```python
from build123d import *

# Parameters (mm, degrees)
F0_W     = 63.5
F0_H     = 63.5
F0_R     = 15.9639
F1_DEPTH = 19.05
F2_R     = 3.175
F3_DEPTH = 34.925


with BuildPart() as f1:
    # F0 (on Front) → F1 (new body, symmetric)
    with BuildSketch(Plane.XZ):
        Rectangle(F0_W, F0_H)
        Circle(F0_R, mode=Mode.SUBTRACT)
    extrude(amount=F1_DEPTH, both=True)

    # F2 (on Right) → F3 (cut, symmetric)
    with BuildSketch(Plane.YZ):
        with Locations((0, 22.225)):
            Circle(F2_R)
        with Locations((0, -22.225)):
            Circle(F2_R)
    extrude(amount=F3_DEPTH, both=True, mode=Mode.SUBTRACT)


solid = f1.part
```
Model file for the job. Use its own axes, mm. Coordinates: 2 decimals unless noted, no trailing zeros. Order: outer loops, then holes, each group sorted by start corner. A loop starts at its lowest first (then second) coordinate and runs counter-clockwise, first axis right, second up. Notation, with made-up numbers: (88, 17) -> (114, 17) arc R33 ccw to (114, 48) -> close; hole circle Ø5 at (51.5, -29.75). An arc over 180 degrees is marked (long way). Answer as a JSON object with one key per item and string values. Group by question number.
1) Pull direction Y, two halves, no side cores. Call faces 1 (the face through (0.444, -0.413, 25.373)), 2 (the face through (-8, 19.05, 15)), 3 (the face through (-31.75, 0, 0)): +Y half, -Y half, draft (parallel to the pull), parting line (faces both ways), or undercut.
2) Cut at A-A, the plane y = 0. Write the cut outline in (x, z), then the cut area to 3 significant figures.
3) Cut at C-C, the plane y = -17. Write the cut outline in (x, z).
4) Cut at D-D, the plane x = 0. Write the cut outline in (y, z) (3 decimals), then the cut area to 3 significant figures.
5) Drill centre lines: L1, parallel to Z at x = 5, y = 0; L2, parallel to Z at x = 11.5, y = 0; L3, parallel to Z at x = 27, y = 2.5. Where is each one in solid material? Low to high.
6) Cut at B-B, the plane z = 0. Write the cut outline in (x, y).
Check values:
{
 "1": {"face 1": "undercut", "face 2": "+Y half", "face 3": "draft"},
 "2": {"outline": "(-31.75, -31.75) -> (31.75, -31.75) -> (31.75, -25.4) -> (-31.75, -25.4) -> close; (-31.75, -19.05) -> (31.75, -19.05) -> (31.75, 19.05) -> (-31.75, 19.05) -> close; (-31.75, 25.4) -> (31.75, 25.4) -> (31.75, 31.75) -> (-31.75, 31.75) -> close; hole circle Ø31.93 at (0, 0)", "area": "2,430 mm²"},
 "3": {"outline": "(-31.75, -31.75) -> (31.75, -31.75) -> (31.75, 31.75) -> (-31.75, 31.75) -> close; hole circle Ø31.93 at (0, 0)"},
 "4": {"outline": "(-19.05, -31.75) -> (19.05, -31.75) -> (19.05, -15.964) -> (-19.05, -15.964) -> close; (-19.05, 15.964) -> (19.05, 15.964) -> (19.05, 31.75) -> (-19.05, 31.75) -> close; hole circle Ø6.35 at (0, -22.225); hole circle Ø6.35 at (0, 22.225)", "area": "1,140 mm²"},
 "5": {"L1": "z = -31.75 to -25.4, -19.05 to -15.16, 15.16 to 19.05, 25.4 to 31.75", "L2": "z = -31.75 to -25.4, -19.05 to -11.07, 11.07 to 19.05, 25.4 to 31.75", "L3": "z = -31.75 to -24.18, -20.27 to 20.27, 24.18 to 31.75"},
 "6": {"outline": "(-31.75, -19.05) -> (-15.96, -19.05) -> (-15.96, 19.05) -> (-31.75, 19.05) -> close; (15.96, -19.05) -> (31.75, -19.05) -> (31.75, 19.05) -> (15.96, 19.05) -> close"}
}
